Print and shaded views of the part. All mm, measured from the part's lowest x, y and z. A direction names the side the tool comes from. Round coordinates to 2 decimals unless told otherwise and drop trailing zeros. Write each loop counter-clockwise with the first axis right and the second up, starting at its lowest first coordinate (ties: lowest second). Pieces come first, ordered by that corner, then holes.
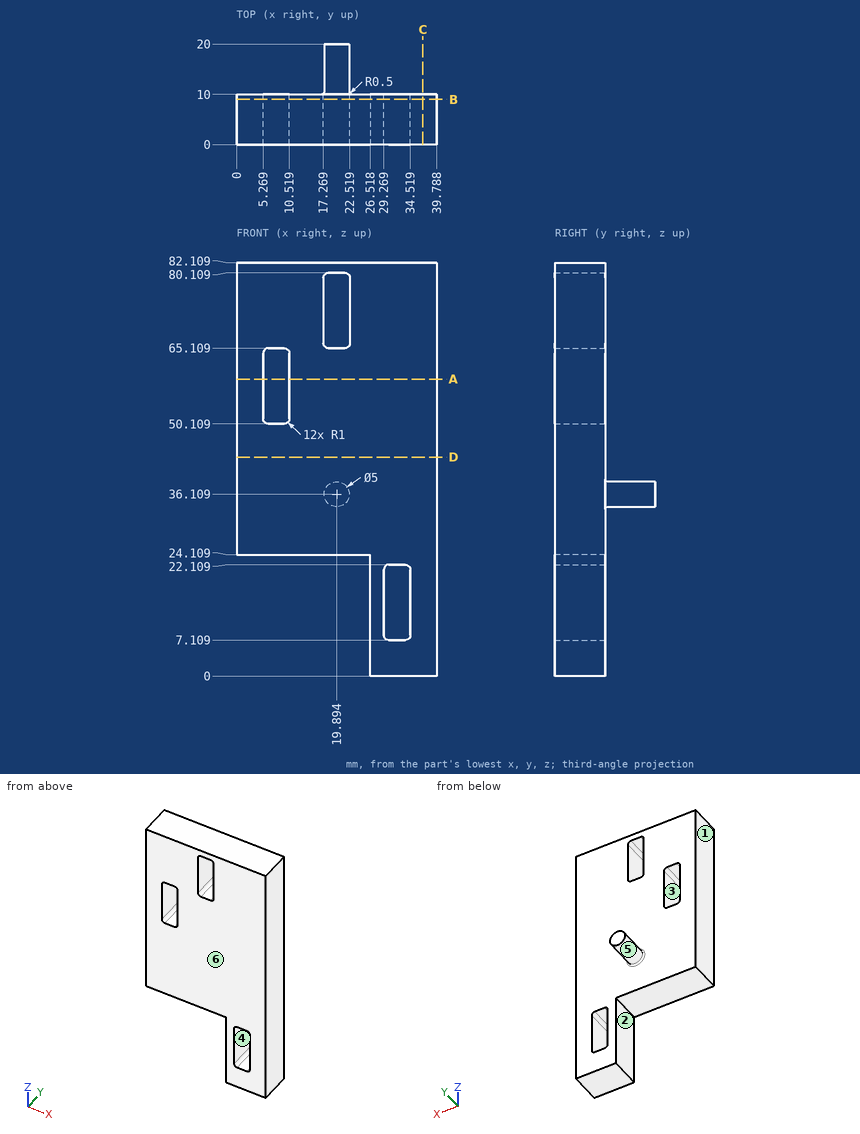
1) Slice it at A-A (z = 59). Write the cut outline in (x, y), plus the area to 3 significant figures.
Results:
outline: (0, 0) - (5.27, 0) - (5.27, 10) - (0, 10) - close; (10.52, 0) - (39.79, 0) - (39.79, 10) - (10.52, 10) - close
area: 345 mm2
2) Slice it at B-B (y = 9). Count the separate pieces of the cut face and the enclosed holes in it, plus the area to 3 significant figures.
Results:
separate pieces: 1
enclosed holes: 3
area: 2,390 mm2
3) Pin check, flat tips, straight feed: pin 1 Ø1 at (x, y) = (32, 3.5) entering from -Z; pin 2 Ø2.5 at (x, y) = (7.5, 6) entering from -Z; pin 3 Ø5 at (y, z) = (7.5, 15) entering from -X; pin 4 Ø3 at (x, z) = (15.5, 62) entering from +Y. Stop position of each tip, or through.
Results:
pin 1: stops at z = 0
pin 2: stops at z = 24.11
pin 3: stops at x = 26.52
pin 4: stops at y = 10
4) Which spindle directions (+Z, -Z, +X, -X, +Y, -Y) get a long thin tool onto all of the face, cutting with end or side? Do the marked faces 1, 2 and 3. Say none if no direction does.
Results:
face 1: +Z, -Z, -X, +Y, -Y
face 2: -Z, -X, +Y, -Y
face 3: +Y, -Y
5) Wall check: L1, parallel to Z at x = 8.5, y = 4.25; L2, parallel to X at y = 6.5, z = 72.5; L3, parallel to Z at x = 21, y = 6.25. Give the ranges that are in metal, low to high.
Results:
L1: z = 24.11 to 50.11, 65.11 to 82.11
L2: x = 0 to 17.27, 22.52 to 39.79
L3: z = 24.11 to 65.11, 80.11 to 82.11
6) Slice it at C-C (x = 37). Write the cut outline in (y, z), plus the area to 3 significant figures.
Results:
outline: (0, 0) - (10, 0) - (10, 82.11) - (0, 82.11) - close
area: 821 mm2
7) Mould opens along X. For the marked faces 4, 5 and 6 say: released by +X, released by -X, zero draft, split by the parting line, or undercut.
Results:
face 4: undercut
face 5: split by the parting line
face 6: zero draft
8) Slice it at D-D (z = 43.5). Write the cut outline in (x, y).
Results:
outline: (0, 0) - (39.79, 0) - (39.79, 10) - (0, 10) - close
